from build123d import *

# Parameters (mm, degrees)
SKETCH_1_R      = 9.65
SKETCH_1_R_2    = 1.65
EXTRUDE_1_DEPTH = 2.6
FILLET_1_R      = 3


with BuildPart() as part:
    # 草图1 → 凸台-拉伸1 (new body)
    with BuildSketch(Plane.XY):
        with BuildLine():
            Line((0, 30), (-5.7, 30))
            Line((-5.7, 30), (-5.7, 10.843085354))
            ThreePointArc((-5.7, 10.843085354), (-12.25, 0), (-5.7, -10.843085354))
            Line((-5.7, -10.843085354), (-5.7, -30))
            Line((-5.7, -30), (0, -30))
            Line((0, -30), (5.7, -30))
            Line((5.7, -30), (5.7, -10.843085354))
            ThreePointArc((5.7, -10.843085354), (12.25, 0), (5.7, 10.843085354))
            Line((5.7, 10.843085354), (5.7, 30))
            Line((5.7, 30), (0, 30))
        make_face()
        Circle(SKETCH_1_R, mode=Mode.SUBTRACT)
        with Locations((0, 26)):
            Circle(SKETCH_1_R_2, mode=Mode.SUBTRACT)
        with Locations((0, -26)):
            Circle(SKETCH_1_R_2, mode=Mode.SUBTRACT)
    extrude(amount=EXTRUDE_1_DEPTH)

    # 圆角1
    fillet_1_edges = [part.edges().sort_by_distance(p)[0] for p in [
        (5.7, -10.843085354, 1.3),
        (-5.7, -10.843085354, 1.3),
        (-5.7, 10.843085354, 1.3),
        (5.7, 10.843085354, 1.3),
    ]]
    fillet(fillet_1_edges, radius=FILLET_1_R)


solid = part.part
Can you work these out from the model? Positions are in its coordinate system, mm. A direction names the side the tool comes from. Coordinates: 2 decimals unless noted, no trailing zeros. Loops run counter-clockwise (first coordinate to the right, second up) from the corner with the lowest first, then second, coordinate; pieces in that order, holes last. Notation, with made-up numbers: (0, 14.5) - (16, 14.5) arc R14 ccw to (16, 25.5) - close; hole circle Ø7 at (-22, -8). An arc over 180 degrees is marked (long way). Answer as a JSON object with one key per item and string values. Group by question number.
Item 1: If we mould it in two halves opening along X, with no side actions, what happens to faces 1 (the face through (6.05, -11.12, 1.32)), 2 (the face through (-0.215, -24.364, 1.282)), 3 (the face through (-8, -6, 0))? For each: released by +X, released by -X, zero draft, split by the parting line, or undercut.
Item 2: If we section it at B-B (y = 0): List the corners of the cut face in (x, z) for me, plus the area to 3 significant figures.
Item 3: If we section it at A-A (x = 0): List the corners of the cut face in (y, z) for me, plus the area to 3 significant figures.
Item 4: If I drill on L1, parallel to Y at x = 0, z = 1.25; L2, parallel to X at y = -13.5, z = 0.75; L3, parallel to Y at x = -1, z = 1.6, over which ranges is the centre line in solid material (lowest first)? Write a range as from..to.
Item 5: For pin 1 (1.3 mm diameter, centred on y = -21, z = 1.5, fed in from -X); pin 2 (1 mm diameter, centred on x = 8.5, z = 2, fed in from -Y); pin 3 (1.5 mm diameter, centred on y = -8, z = 2, fed in from +X), each with a flat end and sliding along its axis, tell me the tip position at first contact or that it passes through.
Item 6: If we section it at C-C (z = 1.35): List the corners of the cut face in (x, y) for me, plus the area to 3 significant figures.
Item 7: On a 3-axis mill with a long thin cutter (end or side, diameter ignored), from which of +Z, -Z, +X, -X, +Y, -Y can I reach the whole of each face in a straight line? I mean faces 4 (the face through (5.7, 21, 1)), 5 (the face through (-5.7, -21, 1)), 6 (the face through (-5.7, 21, 1)), 7 (the face through (5.7, -21, 1)). Say none if no direction works.
Item 8: If we section it at D-D (x = -8): List the corners of the cut face in (y, z) for me, plus the area to 3 significant figures.
Returned:
{
 "1": {"face 1": "released by +X", "face 2": "undercut", "face 3": "zero draft"},
 "2": {"outline": "(-12.25, 0) - (-9.65, 0) - (-9.65, 2.6) - (-12.25, 2.6) - close; (9.65, 0) - (12.25, 0) - (12.25, 2.6) - (9.65, 2.6) - close", "area": "13.5 mm²"},
 "3": {"outline": "(-30, 0) - (-27.65, 0) - (-27.65, 2.6) - (-30, 2.6) - close; (-24.35, 0) - (-9.65, 0) - (-9.65, 2.6) - (-24.35, 2.6) - close; (9.65, 0) - (24.35, 0) - (24.35, 2.6) - (9.65, 2.6) - close; (27.65, 0) - (30, 0) - (30, 2.6) - (27.65, 2.6) - close", "area": "88.7 mm²"},
 "4": {"L1": "y = -30..-27.65, -24.35..-9.65, 9.65..24.35, 27.65..30", "L2": "x = -5.7..5.7", "L3": "y = -30..-27.31, -24.69..-9.6, 9.6..24.69, 27.31..30"},
 "5": {"pin 1": "stops at x = -5.7", "pin 2": "stops at y = -9.28", "pin 3": "stops at x = 9.87"},
 "6": {"outline": "(-6.99, -10.06) arc R3 cw to (-5.7, -12.52) - (-5.7, -30) - (5.7, -30) - (5.7, -12.52) arc R3 cw to (6.99, -10.06) arc R12.25 ccw to (6.99, 10.06) arc R3 cw to (5.7, 12.52) - (5.7, 30) - (-5.7, 30) - (-5.7, 12.52) arc R3 cw to (-6.99, 10.06) arc R12.25 ccw to start; hole circle Ø19.3 at (0, 0); hole circle Ø3.3 at (0, -26); hole circle Ø3.3 at (0, 26)", "area": "579 mm²"},
 "7": {"face 4": "+Z, -Z, +X, +Y", "face 5": "+Z, -Z, -X, -Y", "face 6": "+Z, -Z, -X, +Y", "face 7": "+Z, -Z, +X, -Y"},
 "8": {"outline": "(-9.28, 0) - (-5.4, 0) - (-5.4, 2.6) - (-9.28, 2.6) - close; (5.4, 0) - (9.28, 0) - (9.28, 2.6) - (5.4, 2.6) - close", "area": "20.2 mm²"}
}
